Design review of the part shown in the three views and the two pictorial views. Dimensions are in mm from the part's minimum x, y and z. Coordinates: 2 decimals unless noted, no trailing zeros. Loops run counter-clockwise (first coordinate to the right, second up) from the corner with the lowest first, then second, coordinate; pieces in that order, holes last.
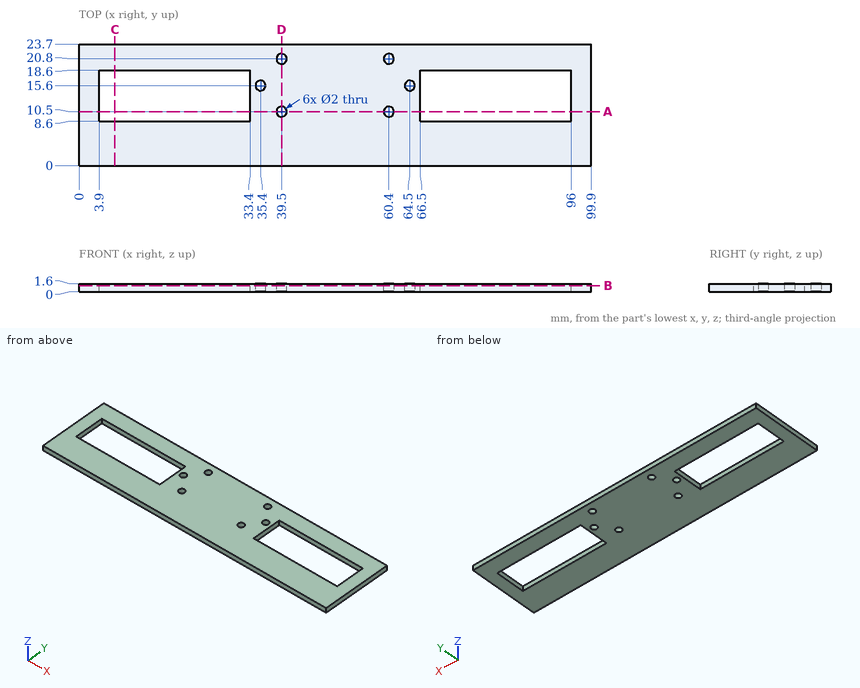
Q1. Wall thickness on probe 1 along Y at (x, z) = (60.4, 1.25); probe 2 along X at (y, z) = (15.6, 1.1); probe 3 along X at (y, z) = (21.5, 0.75): over which ranges is each line inside the solid? List them lowest first.
Q2. Consider section D-D (x = 39.5). State the section outline as (y, z) points.
Q3. Consider section C-C (x = 7). State the section outline as (y, z) points, then the cut area to 3 significant figures.
Q4. Consider section A-A (y = 10.5). State the section outline as (x, z) points.
Q5. Consider section B-B (z = 1.2). Count the separate pieces of the cut face and the enclosed holes in it, then the cut area to 3 significant figures.
Model answer:
1. probe 1: y = 0 to 9.5, 11.5 to 19.8, 21.8 to 23.7
1. probe 2: x = 0 to 3.9, 33.4 to 34.4, 36.4 to 63.5, 65.5 to 66.5, 96 to 99.9
1. probe 3: x = 0 to 38.79, 40.21 to 59.69, 61.11 to 99.9
2. outline: (0, 0) - (9.5, 0) - (9.5, 1.6) - (0, 1.6) - close; (11.5, 0) - (19.8, 0) - (19.8, 1.6) - (11.5, 1.6) - close; (21.8, 0) - (23.7, 0) - (23.7, 1.6) - (21.8, 1.6) - close
3. outline: (0, 0) - (8.6, 0) - (8.6, 1.6) - (0, 1.6) - close; (18.6, 0) - (23.7, 0) - (23.7, 1.6) - (18.6, 1.6) - close
3. area: 21.9 mm2
4. outline: (0, 0) - (3.9, 0) - (3.9, 1.6) - (0, 1.6) - close; (33.4, 0) - (38.5, 0) - (38.5, 1.6) - (33.4, 1.6) - close; (40.5, 0) - (59.4, 0) - (59.4, 1.6) - (40.5, 1.6) - close; (61.4, 0) - (66.5, 0) - (66.5, 1.6) - (61.4, 1.6) - close; (96, 0) - (99.9, 0) - (99.9, 1.6) - (96, 1.6) - close
5. separate pieces: 1
5. enclosed holes: 8
5. area: 1,760 mm2
